Here's the drawing with two shaded views (mm, measured from the low corner). I have some questions. A direction names the side the tool comes from. Coordinates: 2 decimals unless noted, no trailing zeros. Loops run counter-clockwise (first coordinate to the right, second up) from the corner with the lowest first, then second, coordinate; pieces in that order, holes last. Notation, with made-up numbers: (-2, 27) - (24, 27) arc R21 cw to (24, 41) - close; hole circle Ø11 at (60.25, 44). An arc over 180 degrees is marked (long way). Use a Markdown table: item, result.
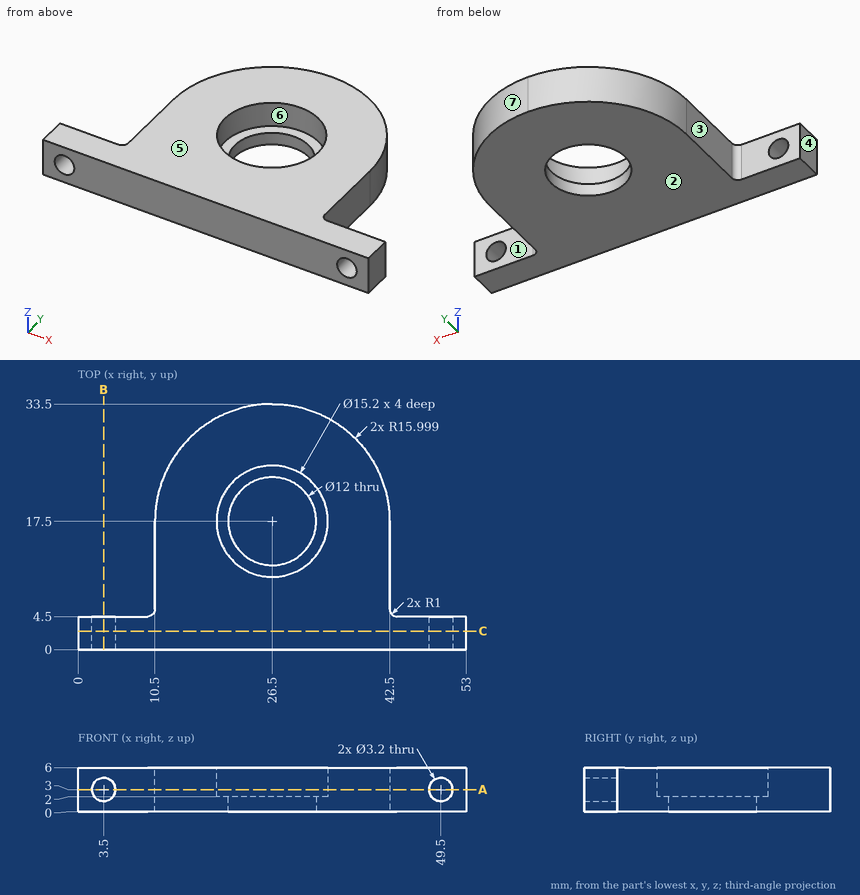
Q1. I want a section at C-C, the plane y = 2.5. Write out the boundary of the cut face in (x, z).
Check values:
| item | result |
|---|---|
| outline | (0, 0) - (53, 0) - (53, 6) - (0, 6) - close; hole circle Ø3.2 at (3.5, 3); hole circle Ø3.2 at (49.5, 3) |
Q2. Will these pins go through, and if not, where does the flat tip stop? P1, Ø3, axis at y = 29, z = 2.5, coming from the -X side; P2, Ø1.8, axis at x = 50, z = 1.5, coming from the +Y side; P3, Ø3, axis at y = 13.5, z = 2, coming from the -X side.
Check values:
| item | result |
|---|---|
| P1 | x = 14.01 |
| P2 | y = 4.5 |
| P3 | x = 10.5 |
Q3. I want a section at A-A, the plane z = 3. Give the number of separate pieces and of enclosed holes in the cut face, then the cut area to 3 significant figures.
Check values:
| item | result |
|---|---|
| separate pieces | 3 |
| enclosed holes | 1 |
| area | 847 mm^2 |
Q4. If we mould it in two halves opening along X, with no side actions, what happens to the marked faces 4, 5, 6 and 7? For each: pulls with the +X half, pulls with the -X half, needs draft (parallel to the pull), parting line crosses it, or undercut.
Check values:
| item | result |
|---|---|
| face 4 | pulls with the -X half |
| face 5 | needs draft |
| face 6 | undercut |
| face 7 | pulls with the +X half |
Q5. Which directions (+Z, -Z, +X, -X, +Y, -Y) give clear straight access to the entire face, cutting with the end or side of a thin tool? Please do the marked faces 1, 2 and 3.
Check values:
| item | result |
|---|---|
| face 1 | +Z, -Z, +X, +Y |
| face 2 | -Z, +X, -X, +Y, -Y |
| face 3 | +Z, -Z, -X, +Y |
Q6. I want a section at B-B, the plane x = 3.5. Write out the boundary of the cut face in (y, z).
Check values:
| item | result |
|---|---|
| outline | (0, 0) - (4.5, 0) - (4.5, 1.4) - (0, 1.4) - close; (0, 4.6) - (4.5, 4.6) - (4.5, 6) - (0, 6) - close |
Q7. Please list where these lines run through material, in increasing order: L1, parallel to X at y = 1.25, z = 3; L2, parallel to Y at x = 9, z = 5.4; L3, parallel to Z at x = 3.5, y = 3. Write a range as from..to.
Check values:
| item | result |
|---|---|
| L1 | 0..1.9, 5.1..47.9, 51.1..53 |
| L2 | 0..4.5 |
| L3 | 0..1.4, 4.6..6 |
